Verification items for the finished model (mm, model axes). Round coordinates to 2 decimals unless told otherwise and drop trailing zeros. Order: outer loops, then holes, each group sorted by start corner. A loop starts at its lowest first (then second) coordinate and runs counter-clockwise, first axis right, second up. Notation, with made-up numbers: M -34,84 L -27,84 A31 cw -27,111 Z; hole C 66,86.5 d8. An arc over 180 degrees is marked long. One line per item, written item: value. Start each with the question number.
Autodesk Inventor part; units mm, degrees
ref_plane "YZ Plane" through (0, 0, 0) normal (1, 0, 0) x (0, 1, 0)
ref_plane "XZ Plane" through (0, 0, 0) normal (0, 1, 0) x (-1, 0, 0)
ref_plane "XY Plane" through (0, 0, 0) normal (0, 0, 1) x (1, 0, 0)
sketch "Sketch1" plane through (0, 0, 0) normal (0, 1, 0) x (-1, 0, 0)
  line L0 (0, 0) -> (45.5, 0)
  line L1 (45.5, 0) -> (45.5, -55)
  line L2 (45.5, -55) -> (0, -55)
  line L3 (0, -55) -> (0, 0)
  dimension "d0" = 45.5
  dimension "d1" = 55
extrude "Extrusion1" add sketch "Sketch1" along normal blind 3
sketch "Sketch2" plane through (0, 3, 0) normal (0, 1, 0) x (1, 0, 0)
  line L0 (-45.5, 55) -> (-45.5, 0)
  line L1 (-45.5, 40) -> (0, 40)
  line L2 (0, 0) -> (0, 55)
  line L3 (0, 55) -> (-45.5, 55)
  circle A0 centre (-6, 34) radius 1
  circle A1 centre (-6, 6) radius 1
  line L4 (-45.5, 0) -> (0, 0)
  line L5 (0, 55) -> (-45.5, 55)
  line L6 (-45.5, 55) -> (-45.5, 52)
  line L7 (-45.5, 52) -> (0, 52)
  line L8 (0, 52) -> (0, 55)
  circle A2 centre (-6, 53.5) radius 0.5
  line L9 (-22.75, 55) -> (-22.75, 53.5)
  circle A3 centre (-39.5, 53.5) radius 0.5
  dimension "d4" = 15
  dimension "d5" = 2
  dimension "d6" = 6
  dimension "d7" = 6
  dimension "d8" = 2
  dimension "d9" = 6
  dimension "d10" = 6
  dimension "d18" = 3
  dimension "d19" = 1
  dimension "d20" = 6
hole "Hole1" at (-6, 3, -6) at (-6, 3, -34) at (-6, 3, -53.5) at (-39.5, 3, -53.5) direction (0, -1, 0) diameter 2 end through all
sketch "Sketch3" plane through (0, 3, 0) normal (0, 1, 0) x (1, 0, 0)
  point P0 (0, 0)
properties part number "SideSupport" material "Wood (Birch)"
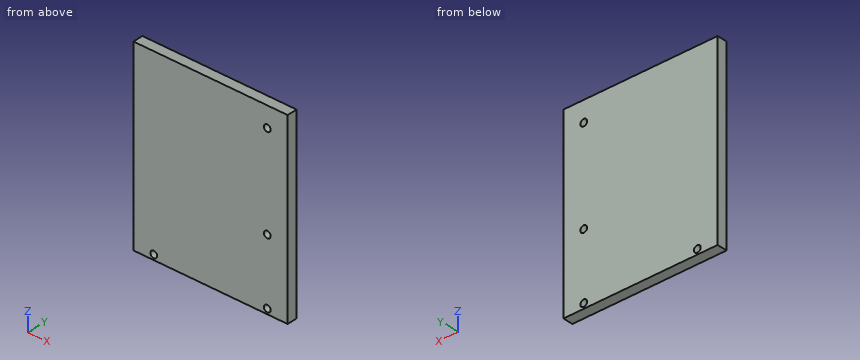
1. Section check A-A (z = -53.5). Record the cut outline in (x, y).
2. Scan lines: line 1 along X through (y, z) = (2.15, -53.5); line 2 along Z through (x, y) = (-6, 1.75); line 3 along X through (y, z) = (2.1, -6). Record each from-to range of solid material in increasing order.
3. Section check C-C (z = -6). Record the cut outline in (x, y), and give its area (4 significant figures).
4. Section check B-B (x = -39.5). Record the cut outline in (y, z), and give its area (3 significant figures).
Geometry check:
1. outline: M -45.5,0 L -40.5,0 L -40.5,3 L -45.5,3 Z; M -38.5,0 L -7,0 L -7,3 L -38.5,3 Z; M -5,0 L 0,0 L 0,3 L -5,3 Z
2. line 1: x = -45.5 to -40.5, -38.5 to -7, -5 to 0
2. line 2: z = -55 to -54.5, -52.5 to -35, -33 to -7, -5 to 0
2. line 3: x = -45.5 to -7, -5 to 0
3. outline: M -45.5,0 L -7,0 L -7,3 L -45.5,3 Z; M -5,0 L 0,0 L 0,3 L -5,3 Z
3. area: 130.5 mm²
4. outline: M 0,-55 L 3,-55 L 3,-54.5 L 0,-54.5 Z; M 0,-52.5 L 3,-52.5 L 3,0 L 0,0 Z
4. area: 159 mm²
